```python
from build123d import *

# Parameters (mm, degrees)
SKETCH1_R           = 38.1
SKETCH1_R_2         = 12.7
BOSS_EXTRUDE1_DEPTH = 25.4


with BuildPart() as part:
    # Sketch1 → Boss-Extrude1 (new body)
    with BuildSketch(Plane.XY):
        Circle(SKETCH1_R)
        Circle(SKETCH1_R_2, mode=Mode.SUBTRACT)
    extrude(amount=BOSS_EXTRUDE1_DEPTH)

    # Cut-Sweep2: sweep along a path in Sketch2
    with BuildLine(Plane(origin=(0, 0, 0), x_dir=(-1, 0, 0), z_dir=(0, 0, -1))) as cut_sweep2_path:
        Line((-14.664696837, 25.4), (-29.329393675, 0))
        Line((-29.329393675, 0), (-14.664696837, -25.4))
        Line((-14.664696837, -25.4), (14.664696837, -25.4))
        Line((14.664696837, -25.4), (29.329393675, 0))
        Line((29.329393675, 0), (14.664696837, 25.4))
        Line((14.664696837, 25.4), (-14.664696837, 25.4))
    # Sketch3 → Cut-Sweep2 (sweep, cut)
    with BuildSketch(Plane(origin=(0, 0, 0), x_dir=(1, 0, 0), z_dir=(0, 1, 0))):
        with BuildLine():
            Line((-35.679393675, 0), (-22.979393675, 0))
            Line((-22.979393675, 0), (-22.979393675, -3.175))
            ThreePointArc((-22.979393675, -3.175), (-23.909329645, -5.42006403), (-26.154393675, -6.35))
            Line((-26.154393675, -6.35), (-32.504393675, -6.35))
            ThreePointArc((-32.504393675, -6.35), (-34.749457705, -5.42006403), (-35.679393675, -3.175))
            Line((-35.679393675, -3.175), (-35.679393675, 0))
        make_face()
    sweep(path=cut_sweep2_path.line, transition=Transition.RIGHT, mode=Mode.SUBTRACT)


solid = part.part
```
The model under review builds one solid part; all positions refer to its coordinate system, in mm. A direction names the side the tool comes from. Coordinates: 2 decimals unless noted, no trailing zeros. Write each loop counter-clockwise with the first axis right and the second up, starting at its lowest first coordinate (ties: lowest second). Pieces come first, ordered by that corner, then holes.
1) Machinability: for faces 4 (the face through (16, 1, 25.4)), 5 (the face through (-23, -6, 6.35)), which of the approach directions +Z, -Z, +X, -X, +Y, -Y give a long, thin tool a straight path to every point of the face, cutting with its end or side? Answer none if there is none.
2) To check wall thickness, follow probe 1 along Y at (x, z) = (0, 18.5); probe 2 along Y at (x, z) = (16, 1.75); probe 3 along Y at (x, z) = (-15.5, 4). State the ranges of each line that lie inside material, in increasing order.
3) The part is to be moulded in two halves that separate along X. For faces 1 (the face through (10, 9, 0)), 2 (the face through (-30.235, -23.183, 12.522)), 3 (the face through (-2.75, -12.4, 12.52)), say which applies: pulls with the +X half, pulls with the -X half, needs draft (parallel to the pull), parting line crosses it, or undercut.
4) Clearance check with flat-ended pins moving along their axes: pin 1 Ø2.5 at (x, z) = (2, 1.5) entering from -Y; pin 2 Ø2.5 at (x, z) = (-4, 1) entering from +Y; pin 3 Ø4 at (x, y) = (26, 28.5) entering from +Z; pin 4 Ø1.5 at (y, z) = (19.5, 20.5) entering from +X. State where each tip first meets the part, or that it passes through.
5) We need section A-A on z = 20.5. State the section outline as (x, y) points, then the cut area to 3 significant figures.
Answer list:
1. face 4: +Z, +X, -X, +Y, -Y
1. face 5: -Z
2. probe 1: y = -38.1 to -12.7, 12.7 to 38.1
2. probe 2: y = -34.58 to -30.9, -12.09 to 12.09, 30.9 to 34.58
2. probe 3: y = -34.8 to -30.8, -13.14 to 13.14, 30.8 to 34.8
3. face 1: needs draft
3. face 2: parting line crosses it
3. face 3: undercut
4. pin 1: stops at y = -38.09
4. pin 2: stops at y = 38
4. pin 3: stops at z = 25.4
4. pin 4: stops at x = 33.17
5. outline: circle Ø76.2 at (0, 0); hole circle Ø25.4 at (0, 0)
5. area: 4,050 mm2
